Part model, mm, in its own coordinate system. Give positions to 0.01 mm unless a question says otherwise; leave off trailing zeros. Order: outer loops, then holes, each group sorted by start corner. A loop starts at its lowest first (then second) coordinate and runs counter-clockwise, first axis right, second up. Notation, with made-up numbers: M 37,63.5 L 62,63.5 A18 ccw 62,86.5 Z; hole C 62,8 d3. An arc over 180 degrees is marked long. Return JSON: item names as keys, results as strings.
from build123d import *

# Parameters (mm, degrees)
SKETCH1_R                  = 1.1
SKETCH1_W                  = 22
SKETCH1_H                  = 40
SKETCH1_W_2                = 6
SKETCH1_H_2                = 8
BOSS_EXTRUDE1_DEPTH        = 6
F_1_6_1_6_DIAMETER_HOLE3_D = 1.6
BOSS_EXTRUDE2_DEPTH        = 6
FILLET1_R                  = 2
F_2_2_2_2_DIAMETER_HOLE1_D = 2.2
F_4_0MM_DOWEL_HOLE1_D      = 4.5
F_2_0MM_DOWEL_HOLE1_D      = 2.2


with BuildPart() as part:
    # Sketch1 → Boss-Extrude1 (new body)
    with BuildSketch(Plane(origin=(0, 0, 0), x_dir=(1, 0, 0), z_dir=(0, 1, 0))):
        Polygon((14.366669751, 50.883801944), (36.883330249, 37.883801944), (36.883330249, -37.883801944), (14.366669751, -50.883801944), (5.706415713, -45.883801944), (5.706415713, -28), (-25.269237886, -28), (-51.25, -13), (-51.25, 13), (-25.269237886, 28), (5.706415713, 28), (5.706415713, 45.883801944), align=None)
        with Locations(Location((15.705771366, 45.203193978, 0), (0, 0, 270))):
            Circle(SKETCH1_R, mode=Mode.SUBTRACT)
        with Locations(Location((31.294228634, 36.203193978, 0), (0, 0, 270))):
            Circle(SKETCH1_R, mode=Mode.SUBTRACT)
        with Locations(Location((31.294228634, -36.203193978, 0), (0, 0, 270))):
            Circle(SKETCH1_R, mode=Mode.SUBTRACT)
        with Locations(Location((15.705771366, -45.203193978, 0), (0, 0, 270))):
            Circle(SKETCH1_R, mode=Mode.SUBTRACT)
        with Locations(Location((-47, 9, 0), (0, 0, 270))):
            Circle(SKETCH1_R, mode=Mode.SUBTRACT)
        with Locations(Location((-47, -9, 0), (0, 0, 270))):
            Circle(SKETCH1_R, mode=Mode.SUBTRACT)
        with Locations((-6.25, 0)):
            Rectangle(SKETCH1_W, SKETCH1_H, mode=Mode.SUBTRACT)
        with Locations((29.633330249, 0)):
            Rectangle(SKETCH1_W_2, SKETCH1_H_2, mode=Mode.SUBTRACT)
    extrude(amount=BOSS_EXTRUDE1_DEPTH)

    # Ø1.6 (1.6) Diameter Hole3 (through all)
    with Locations(Plane(origin=(-6.25, 0, 22.5), x_dir=(0, 0, -1), z_dir=(0, -1, 0))):
        with Locations((0, 0), (45, 0)):
            Hole(F_1_6_1_6_DIAMETER_HOLE3_D / 2)

    # Sketch9 → Boss-Extrude2 (add)
    with BuildSketch(Plane.XZ):
        with BuildLine():
            Line((36.883330249, -9), (36.883330249, -15))
            ThreePointArc((36.883330249, -15), (38.383330249, -14.598076211), (39.481406461, -13.5))
            ThreePointArc((39.481406461, -13.5), (39.883330249, -12), (39.481406461, -10.5))
            ThreePointArc((39.481406461, -10.5), (38.383330249, -9.401923789), (36.883330249, -9))
        make_face()
        with BuildLine():
            Line((36.883330249, -6), (36.883330249, -9))
            ThreePointArc((36.883330249, -9), (38.383330249, -9.401923789), (39.481406461, -10.5))
            Line((39.481406461, -10.5), (36.883330249, -6))
        make_face()
        with BuildLine():
            Line((36.883330249, -15), (36.883330249, -18))
            Line((36.883330249, -18), (39.481406461, -13.5))
            ThreePointArc((39.481406461, -13.5), (38.383330249, -14.598076211), (36.883330249, -15))
        make_face()
        with BuildLine():
            ThreePointArc((39.481406461, 10.5), (39.883330249, 12), (39.481406461, 13.5))
            ThreePointArc((39.481406461, 13.5), (38.383330249, 14.598076211), (36.883330249, 15))
            Line((36.883330249, 15), (36.883330249, 9))
            ThreePointArc((36.883330249, 9), (38.383330249, 9.401923789), (39.481406461, 10.5))
        make_face()
        with BuildLine():
            Line((36.883330249, 6), (39.481406461, 10.5))
            ThreePointArc((39.481406461, 10.5), (38.383330249, 9.401923789), (36.883330249, 9))
            Line((36.883330249, 9), (36.883330249, 6))
        make_face()
        with BuildLine():
            ThreePointArc((36.883330249, 15), (38.383330249, 14.598076211), (39.481406461, 13.5))
            Line((39.481406461, 13.5), (36.883330249, 18))
            Line((36.883330249, 18), (36.883330249, 15))
        make_face()
    extrude(amount=-BOSS_EXTRUDE2_DEPTH)

    # Fillet1
    fillet1_edges = [part.edges().sort_by_distance(p)[0] for p in [
        (32.633330249, 3, 4),
        (32.633330249, 3, -4),
        (26.633330249, 3, -4),
        (26.633330249, 3, 4),
    ]]
    fillet(fillet1_edges, radius=FILLET1_R)

    # Ø2.2 (2.2) Diameter Hole1 (through all)
    with Locations(Plane(origin=(20.133330249, 6, -12), x_dir=(0, 0, 1), z_dir=(0, 1, 0))):
        with Locations((0, 0), (24, 0)):
            Hole(F_2_2_2_2_DIAMETER_HOLE1_D / 2)

    # Ø4.0mm Dowel Hole1 (through all)
    with Locations(Plane(origin=(31.883330249, 6, -12), x_dir=(0, 0, 1), z_dir=(0, 1, 0))):
        with Locations((0, 0), (24, 0)):
            Hole(F_4_0MM_DOWEL_HOLE1_D / 2)

    # Ø2.0mm Dowel Hole1 (through all)
    with Locations(Plane(origin=(-31.25, 6, -15), x_dir=(0, 0, 1), z_dir=(0, 1, 0))):
        with Locations((0, 0), (30, 0), (30, 40), (0, 40)):
            Hole(F_2_0MM_DOWEL_HOLE1_D / 2)


solid = part.part
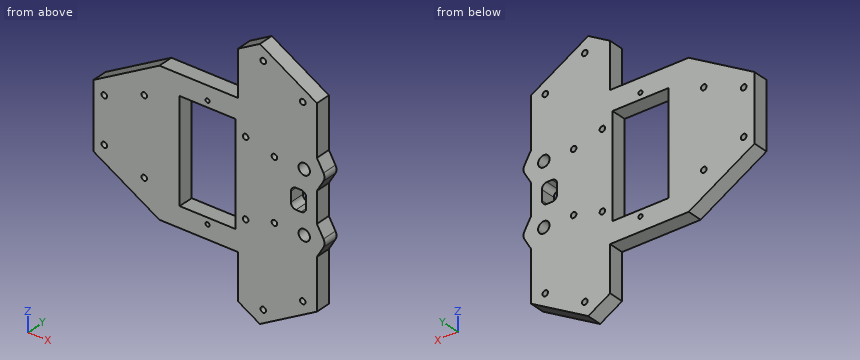
Q1. Band-saw the part on A-A (x = -47). Give the cut face in (y, z).
Established:
{"outline": "M 0,-15.45 L 6,-15.45 L 6,-10.1 L 0,-10.1 Z; M 0,-7.9 L 6,-7.9 L 6,7.9 L 0,7.9 Z; M 0,10.1 L 6,10.1 L 6,15.45 L 0,15.45 Z"}
Q2. Pin check, flat tips, straight feed: pin 1 (1.8 mm diameter, centred on y = 3, z = -30, fed in from +X); pin 2 (8 mm diameter, centred on x = -31, z = 15, fed in from -Y); pin 3 (1.5 mm diameter, centred on y = 4, z = -39.5, fed in from -X); pin 4 (1.8 mm diameter, centred on x = -8.5, y = 3, fed in from -Z). Stop position of each tip, or through.
Established:
{"pin 1": "stops at x = 36.88", "pin 2": "stops at y = 0", "pin 3": "stops at x = 5.71", "pin 4": "stops at z = -28"}
Q3. Band-saw the part on C-C (z = 32.5). Give the cut face in (x, y).
Established:
{"outline": "M 5.71,0 L 36.88,0 L 36.88,6 L 5.71,6 Z"}
Q4. Band-saw the part on B-B (y = 2.3). Give the number of separate pieces and of enclosed holes in the cut face, then the cut area to 3 significant figures.
Established:
{"separate pieces": "1", "enclosed holes": "18", "area": "4,670 mm²"}
Q5. Probe line 1 along X through (y, z) = (2.5, 1); line 2 along X through (y, z) = (3.5, -12); line 3 along Z through (x, y) = (31.5, 3.7). List the from-to ranges inside material, lowest first.
Established:
{"line 1": "x = -51.25 to -17.25, 4.75 to 26.63, 32.63 to 36.88", "line 2": "x = -51.25 to -17.25, 4.75 to 19.03, 21.23 to 29.63, 34.13 to 39.88", "line 3": "z = -40.99 to -37.28, -35.12 to -14.22, -9.78 to -3.8, 3.8 to 9.78, 14.22 to 35.12, 37.28 to 40.99"}
Q6. Band-saw the part on D-D (x = -20). Give the cut face in (y, z).
Established:
{"outline": "M 0,-28 L 6,-28 L 6,28 L 0,28 Z"}
